from build123d import *

# Parameters (mm, degrees)
F0_W     = 66.5
F0_H     = 35
F0_W_2   = 65
F2_R     = 30
F3_DEPTH = 140
F4_R     = 30
F5_DEPTH = 140


with BuildPart() as f1:
    # F0 (on Front) → F1 (revolve)
    with BuildSketch(Plane.XZ):
        with Locations((-165.878672, 17.5)):
            Rectangle(F0_W, F0_H)
        Polygon((-132.628672, 35), (-132.628672, 0), (213.871328, 0), (213.871328, 35), (213.871328, 45), (-132.628672, 45), align=None)
        with Locations((246.371328, 17.5)):
            Rectangle(F0_W_2, F0_H)
    revolve(axis=Axis((40.621328, 0, 0), (1, 0, 0)))

    # F2 (on face) → F3 (join)
    with BuildSketch(Plane(origin=(-199.128672, 0, 0), x_dir=(0, -1, 0), z_dir=(-1, 0, 0))):
        Circle(F2_R)
    extrude(amount=F3_DEPTH)

    # F4 (on face) → F5 (join)
    with BuildSketch(Plane.YZ.offset(278.871328)):
        Circle(F4_R)
    extrude(amount=F5_DEPTH)


solid = f1.part
The listing builds one solid part. Answer for the finished solid, in the listing's coordinates (mm). A direction names the side the tool comes from. Give positions to 0.01 mm unless a question says otherwise; leave off trailing zeros. Loops run counter-clockwise (first coordinate to the right, second up) from the corner with the lowest first, then second, coordinate; pieces in that order, holes last. Notation, with made-up numbers: (46.25, 40.5) - (55.25, 40.5) arc R31 ccw to (55.25, 66.5) - close; hole circle Ø10 at (56, 64.5). An arc over 180 degrees is marked (long way). Answer as a JSON object with one key per item and string values.
1. A cutting plane is placed at A-A (y = 0). Write down the section's boundary in (x, z), then the cut area to 3 significant figures.
Determined:
{"outline": "(-339.13, -30) - (-199.13, -30) - (-199.13, -35) - (-132.63, -35) - (-132.63, -45) - (213.87, -45) - (213.87, -35) - (278.87, -35) - (278.87, -30) - (418.87, -30) - (418.87, 30) - (278.87, 30) - (278.87, 35) - (213.87, 35) - (213.87, 45) - (-132.63, 45) - (-132.63, 35) - (-199.13, 35) - (-199.13, 30) - (-339.13, 30) - close", "area": "57,200 mm²"}
2. For faces 1 (the flat face through (-132.629, 26.5, 23.1)), 2 (the flat face through (278.871, -16, -26)), 3 (the flat face through (-339.129, 0, 0)), determine the directions among +Z, -Z, +X, -X, +Y, -Y from which every point of the face is accessible in a straight line to the end or side of a thin tool.
Determined:
{"face 1": "-X", "face 2": "+X", "face 3": "+Z, -Z, -X, +Y, -Y"}
3. A cutting plane is placed at D-D (x = -59). Write down the section's boundary in (y, z).
Determined:
{"outline": "circle Ø90 at (0, 0)"}
4. Find the intervals of material crossed by L1, parallel to X at y = 8, z = -34.5; L2, parallel to Z at x = -222, y = 2; L3, parallel to X at y = -30, z = -4, in increasing order. Write a range as [from, to].
Determined:
{"L1": "[-132.63, 213.87]", "L2": "[-29.93, 29.93]", "L3": "[-199.13, 278.87]"}
5. A cutting plane is placed at C-C (x = -217). Write down the section's boundary in (y, z), then the cut area to 3 significant figures.
Determined:
{"outline": "circle Ø60 at (0, 0)", "area": "2,830 mm²"}
6. Flat-ended cylindrical pins translate along their axes: pin 1 Ø8 at (x, z) = (-180, 6) entering from +Y; pin 2 Ø12 at (y, z) = (24.5, 32.5) entering from +X; pin 3 Ø6 at (y, z) = (24, -35) entering from -X. Find the tip coordinate at first contact, or state that the pin passes through.
Determined:
{"pin 1": "y = 34.94", "pin 2": "x = 278.87", "pin 3": "x = -132.63"}
